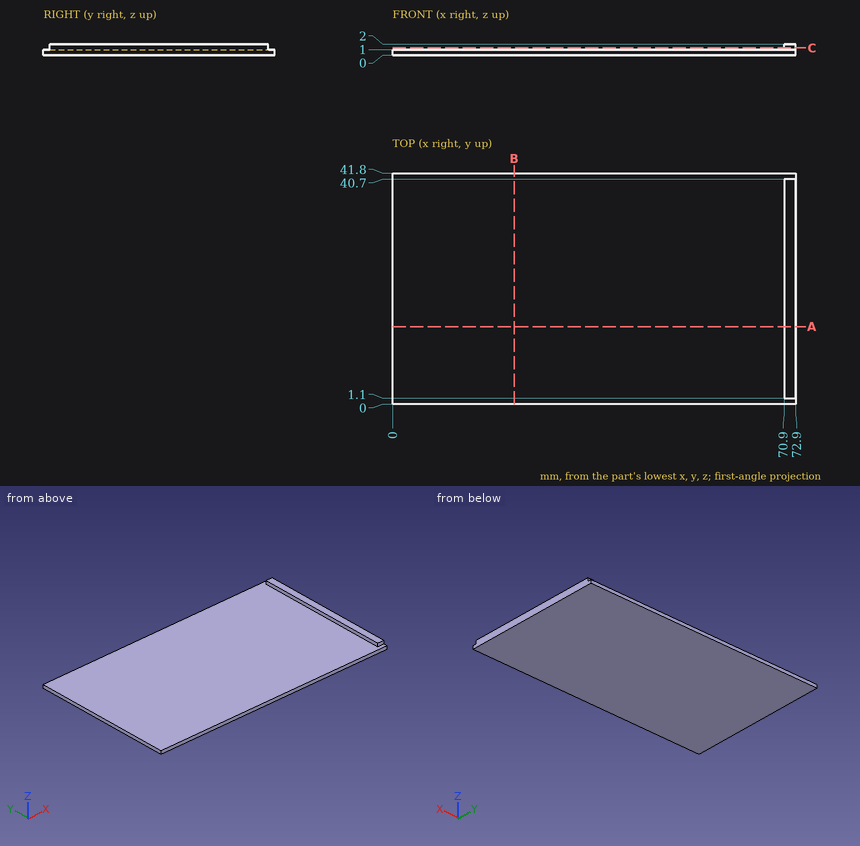
The figure shows three views and two pictorial views of one solid part (mm, origin at its lowest corner). Answer the questions. Give positions to 0.01 mm unless a question says otherwise; leave off trailing zeros. Write each loop counter-clockwise with the first axis right and the second up, starting at its lowest first coordinate (ties: lowest second). Pieces come first, ordered by that corner, then holes.
Q1. The part is cut by section A-A on y = 14. Give the vertices of the cut face in (x, z).
Answer:
outline: (0, 0) - (72.9, 0) - (72.9, 2) - (70.9, 2) - (70.9, 1) - (0, 1) - close
Q2. The part is cut by section B-B on x = 22. Give the vertices of the cut face in (y, z), and give its area (3 significant figures).
Answer:
outline: (0, 0) - (41.8, 0) - (41.8, 1) - (0, 1) - close
area: 41.8 mm2
Q3. The part is cut by section C-C on z = 1.3. Give the vertices of the cut face in (x, y), and give its area (3 significant figures).
Answer:
outline: (70.9, 1.1) - (72.9, 1.1) - (72.9, 40.7) - (70.9, 40.7) - close
area: 79.2 mm2
Q4. Straight lines are drawn through the part: L1, parallel to Z at x = 49.5, y = 32.5; L2, parallel to X at y = 25.5, z = 1.6. For each, find the intervals that lie inside material, in ascending order.
Answer:
L1: z = 0 to 1
L2: x = 70.9 to 72.9
Q5. Given pin 1 (12 mm diameter, centred on x = 21.5, y = 17.5, fed in from +Z); pin 2 (0.5 mm diameter, centred on x = 71.5, z = 1.5, fed in from +Y); pin 3 (0.8 mm diameter, centred on y = 27.5, z = 1.5, fed in from -X); pin 4 (12 mm diameter, centred on x = 62.5, y = 30.5, fed in from -Z), each flat-ended and moving along its own axis, determine where each tip first touches the part or whether it passes through.
Answer:
pin 1: stops at z = 1
pin 2: stops at y = 40.7
pin 3: stops at x = 70.9
pin 4: stops at z = 0
